Here's how the part is built. I have some questions about the finished solid (model axes, mm). Face numbers are marked on the shaded views. A direction names the side the tool comes from. Give positions to 0.01 mm unless a question says otherwise; leave off trailing zeros. Loops run counter-clockwise (first coordinate to the right, second up) from the corner with the lowest first, then second, coordinate; pieces in that order, holes last. Notation, with made-up numbers: (-14, -8.5) - (-8, -8.5) arc R32 cw to (-8, 21.5) - close; hole circle Ø3 at (3.5, 50). An arc over 180 degrees is marked (long way). Return JSON: item names as keys, results as strings. Group by question number.
(1) I need wall thicknesses on probe 1 along Y at (x, z) = (0, 3.05); probe 2 along X at (y, z) = (0, 3.1); probe 3 along X at (y, z) = (0, 2.8). Which ranges of each line are inside material? Lowest first, please. Write a range as [from, to].
(2) If we mould it in two halves opening along X, with no side actions, what happens to the marked faces 1, 2 and 3? For each: released by +X, released by -X, zero draft, split by the parting line, or undercut.
(3) If we section it at B-B (y = 0): State how many separate pieces and enclosed holes the cut face has, then the cut area to 3 significant figures.
(4) On a 3-axis mill with a long thin cutter (end or side, diameter ignored), from which of +Z, -Z, +X, -X, +Y, -Y can I reach the whole of each face in a straight line? I mean the marked faces 4 and 5. Say none if no direction works.
(5) For P1, Ø1.5, axis at x = 10.5, z = 1.5, coming from the -Y side; P2, Ø1.5, axis at x = -12.5, z = 2.5, coming from the +Y side; P3, Ø1.5, axis at y = 7, z = 2.5, coming from the -X side, each with a flat end and sliding along its axis, tell me the tip position at first contact or that it passes through.
(6) If we section it at A-A (x = -5): Please give me the cut outline in (y, z).
```python
from build123d import *

# Parameters (mm, degrees)
PAD_DEPTH       = 3.5
FILLET_R        = 1
POCKET_DEPTH    = 1
SKETCH007_W     = 3
SKETCH007_H     = 1
POCKET001_DEPTH = 2.501
SKETCH008_W     = 8.5
SKETCH008_H     = 2.5
POCKET002_DEPTH = 1
SKETCH009_W     = 1
SKETCH009_H     = 1
POCKET003_DEPTH = 5
SKETCH010_W     = 10.5
SKETCH010_H     = 1
POCKET004_DEPTH = 1.5
SKETCH001_W     = 4.2
SKETCH001_H     = 4.2
POCKET005_DEPTH = 3
SKETCH006_W     = 4
SKETCH006_H     = 1
POCKET006_DEPTH = 0.5


with BuildPart() as part:
    # Sketch → Pad (new body)
    with BuildSketch(Plane.XY):
        with BuildLine():
            ThreePointArc((-7.5, 10), (-17.5, 0), (-7.5, -10))
            Line((-7.5, -10), (7.5, -10))
            ThreePointArc((7.5, -10), (17.5, 0), (7.5, 10))
            Line((-7.5, 10), (7.5, 10))
        make_face()
    extrude(amount=PAD_DEPTH)

    # Fillet
    fillet_edges = [part.edges().sort_by_distance(p)[0] for p in [
        (0, 10, 3.5),
        (0, -10, 3.5),
        (17.5, 0, 3.5),
        (-17.5, 0, 3.5),
    ]]
    fillet(fillet_edges, radius=FILLET_R)

    # Sketch003 → Pocket (cut)
    with BuildSketch(Plane.XY.offset(3.5)):
        with BuildLine():
            ThreePointArc((-2.8, -1.65), (3.25, 0), (-2.8, 1.65))
            Line((-2.8, 1.65), (-2.8, -1.65))
        make_face()
    extrude(amount=-POCKET_DEPTH, mode=Mode.SUBTRACT)

    # Sketch007 → Pocket001 (cut, through all)
    with BuildSketch(Plane.XY.offset(2.5)):
        Rectangle(SKETCH007_W, SKETCH007_H)
    extrude(amount=-POCKET001_DEPTH, mode=Mode.SUBTRACT)

    # Sketch008 → Pocket002 (cut)
    with BuildSketch(Plane.XY.offset(3.5)):
        with Locations((0, -6.25)):
            Rectangle(SKETCH008_W, SKETCH008_H)
    extrude(amount=-POCKET002_DEPTH, mode=Mode.SUBTRACT)

    # Sketch009 → Pocket003 (cut)
    with BuildSketch(Plane.XY.offset(2.5)):
        with Locations((-3.75, -6.25)):
            Rectangle(SKETCH009_W, SKETCH009_H)
        with Locations((3.75, -6.25)):
            Rectangle(SKETCH009_W, SKETCH009_H)
    extrude(amount=-POCKET003_DEPTH, mode=Mode.SUBTRACT)

    # Sketch010 → Pocket004 (cut)
    with BuildSketch(Plane(origin=(0, 0, 0), x_dir=(1, 0, 0), z_dir=(0, 0, -1))):
        Polygon((3.643237, 5.75), (11.696618, -0.397441), (12.303382, 0.397441), (4.25, 6.544883), align=None)
        with Locations((-6.75, 0)):
            Rectangle(SKETCH010_W, SKETCH010_H)
        Polygon((-3.25, 5.75), (0, 5.75), (0, 0.5), (1.5, 0.5), (1.5, 6.75), (-3.25, 6.75), align=None)
    extrude(amount=-POCKET004_DEPTH, mode=Mode.SUBTRACT)

    # Sketch001 → Pocket005 (cut)
    with BuildSketch(Plane.XY.offset(3.5)):
        with Locations((-12.1, 0)):
            Rectangle(SKETCH001_W, SKETCH001_H)
        with Locations((12.1, 0)):
            Rectangle(SKETCH001_W, SKETCH001_H)
    extrude(amount=-POCKET005_DEPTH, mode=Mode.SUBTRACT)

    # Sketch006 → Pocket006 (cut)
    with BuildSketch(Plane.XY.offset(3.5)):
        with Locations((-6, 0)):
            Rectangle(SKETCH006_W, SKETCH006_H)
        Polygon((4, 0.5), (5.5, 0.5), (5.5, 2), (6.5, 2), (6.5, 0.5), (8, 0.5), (8, -0.5), (6.5, -0.5), (6.5, -2), (5.5, -2), (5.5, -0.5), (4, -0.5), align=None)
    extrude(amount=-POCKET006_DEPTH, mode=Mode.SUBTRACT)


solid = part.part
```
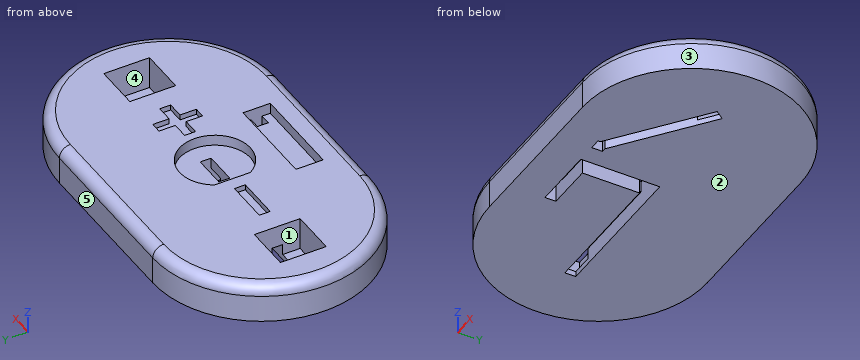
Values:
{
 "1": {"probe 1": "[-9.84, -7.5], [-5, -3.25], [3.25, 9.84]", "probe 2": "[-17.3, -14.2], [-10, -8], [-4, -2.8], [3.25, 4], [8, 10], [14.2, 17.3]", "probe 3": "[-17.45, -14.2], [-10, -2.8], [3.25, 10], [14.2, 17.45]"},
 "2": {"face 1": "undercut", "face 2": "zero draft", "face 3": "released by +X"},
 "3": {"separate pieces": "4", "enclosed holes": "0", "area": "65.2 mm2"},
 "4": {"face 4": "+Z", "face 5": "+Z, -Z, +X, -X, +Y"},
 "5": {"P1": "y = -9.74", "P2": "y = 9.05", "P3": "x = -15.31"},
 "6": {"outline": "(-10, 0) - (-0.5, 0) - (-0.5, 1.5) - (0.5, 1.5) - (0.5, 0) - (10, 0) - (10, 2.5) arc R1 ccw to (9, 3.5) - (0.5, 3.5) - (0.5, 3) - (-0.5, 3) - (-0.5, 3.5) - (-9, 3.5) arc R1 ccw to (-10, 2.5) - close"}
}
